```python
from build123d import *

# Parameters (mm, degrees)
BOSS_EXTRUDE1_DEPTH = 6.75
SKETCH3_R           = 8
CUT_EXTRUDE2_DEPTH  = 0.75
SKETCH4_W           = 27
SKETCH4_H           = 2
CUT_EXTRUDE3_DEPTH  = 9
FILLET1_R           = 4


with BuildPart() as part:
    # Sketch1 → Boss-Extrude1 (new body)
    with BuildSketch(Plane.XY):
        with BuildLine():
            Line((-27, 0), (0, 0))
            Line((0, 0), (0, 12.5))
            Line((0, 12.5), (-7.5, 12.5))
            ThreePointArc((-7.5, 12.5), (-13.5, 6.5), (-19.5, 12.5))
            Line((-19.5, 12.5), (-27, 12.5))
            Line((-27, 12.5), (-27, 0))
        make_face()
    extrude(amount=BOSS_EXTRUDE1_DEPTH)

    # Sketch3 → Cut-Extrude2 (cut)
    with BuildSketch(Plane(origin=(0, 0, 0), x_dir=(-1, 0, 0), z_dir=(0, 0, -1))):
        with Locations((13.5, 12.5)):
            Circle(SKETCH3_R)
    extrude(amount=-CUT_EXTRUDE2_DEPTH, mode=Mode.SUBTRACT)

    # Sketch4 → Cut-Extrude3 (cut)
    with BuildSketch(Plane.XY.offset(6.75)):
        with Locations((-13.5, 11.5)):
            Rectangle(SKETCH4_W, SKETCH4_H)
    extrude(amount=-CUT_EXTRUDE3_DEPTH, mode=Mode.SUBTRACT)

    # Fillet1
    fillet1_edges = [part.edges().sort_by_distance(p)[0] for p in [
        (-27, 10.5, 3.375),
        (0, 10.5, 3.375),
    ]]
    fillet(fillet1_edges, radius=FILLET1_R)


solid = part.part
```
Here's how the part is built. I have some questions about the finished solid (model axes, mm). A direction names the side the tool comes from. Give positions to 0.01 mm unless a question says otherwise; leave off trailing zeros. Loops run counter-clockwise (first coordinate to the right, second up) from the corner with the lowest first, then second, coordinate; pieces in that order, holes last. Notation, with made-up numbers: M -31.5,63.5 L -6.5,63.5 A20 ccw -6.5,75.5 Z; hole C 74.5,-21.75 d6. An arc over 180 degrees is marked long. Put each result on its own line as item: value. Start each with the question number.
(1) I want a section at D-D on y = 4.75. Please give me the cut outline in (x, z).
(2) I need wall thicknesses on line 1 along X through (y, z) = (7, 5.75); line 2 along Y through (x, z) = (-13.5, 6); line 3 along X through (y, z) = (9, 4.5). Which ranges of each line are inside material? Lowest first, please. Write a range as [from, to].
(3) Will this pin go through, and if not, where does the flat tip stop? pin 1 Ø1.5 at (x, z) = (-17, 4.5) entering from +Y.
(4) I want a section at C-C on x = -14. Please give me the cut outline in (y, z).
(5) For faces 4 (the cylindrical face through (-13.4, 4.5, 0.4)), 5 (the cylindrical face through (-13.4, 6.5, 3.7)), which set-ups out of +Z, -Z, +X, -X, +Y, -Y let a thin tool reach every point of the face, with its end or its side?
(6) I want a section at A-A on z = 5. Please give me the cut outline in (x, y), then the cut area to 3 significant figures.
(7) I want a section at B-B on y = 6.75. Please give me the cut outline in (x, z).
(8) If we mould it in two halves opening along X, with no side actions, what happens to faces 1 (the cylindrical face through (-1.141, 9.297, 3.328)), 2 (the flat face through (-13, 6, 0.75)), 3 (the flat face through (-21, 10.5, 3))? For each: +X half, -X half, draft (parallel to the pull), parting line (faces both ways), or undercut.
Answer block:
1. outline: M -27,0 L -15.48,0 L -15.48,0.75 L -11.52,0.75 L -11.52,0 L 0,0 L 0,6.75 L -27,6.75 Z
2. line 1: [-26.97, -15.9], [-11.1, -0.03]
2. line 2: [0, 6.5]
2. line 3: [-26.12, -18.37], [-8.63, -0.88]
3. pin 1: y = 8.26
4. outline: M 0,0 L 4.52,0 L 4.52,0.75 L 6.52,0.75 L 6.52,6.75 L 0,6.75 Z
5. face 4: -Z, +Y
5. face 5: +Z, -Z, +Y
6. outline: M -27,0 L 0,0 L 0,6.5 A4 ccw -4,10.5 L -7.84,10.5 A6 cw -19.16,10.5 L -23,10.5 A4 ccw -27,6.5 Z
6. area: 244 mm^2
7. outline: M -26.99,0 L -19.06,0 L -19.06,0.75 L -15.21,0.75 L -15.21,6.75 L -26.99,6.75 Z; M -11.79,0.75 L -7.94,0.75 L -7.94,0 L -0.01,0 L -0.01,6.75 L -11.79,6.75 Z
8. face 1: +X half
8. face 2: undercut
8. face 3: draft
